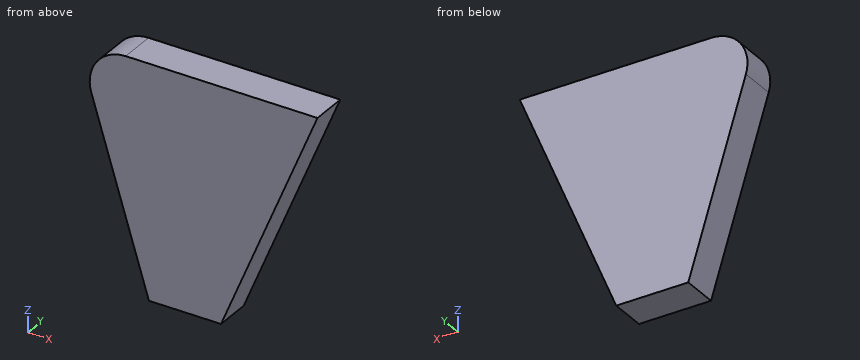
from build123d import *

# Parameters (mm, degrees)
F0_W     = 20
F0_H     = 32.335784
F1_DEPTH = 5
F3_DEPTH = 25
F4_R     = 5


with BuildPart() as f1:
    # F0 (on Front) → F1 (new body)
    with BuildSketch(Plane.XZ):
        with Locations((10, 16.167892)):
            Rectangle(F0_W, F0_H)
        Polygon((20, 32.335784), (20, 0), (33.39392, 32.335784), align=None)
    extrude(amount=F1_DEPTH)

    # F2 (on face) → F3 (cut)
    with BuildSketch(Plane.XZ.offset(5)):
        Polygon((10, 0), (0, 32.335784), (0, 0), align=None)
    extrude(amount=-F3_DEPTH, mode=Mode.SUBTRACT)

    # F4
    f4_edges = [f1.edges().sort_by_distance(p)[0] for p in [
        (0, -2.5, 32.335784),
    ]]
    fillet(f4_edges, radius=F4_R)


solid = f1.part
Can you work these out from the model? Positions are in its coordinate system, mm. Coordinates: 2 decimals unless noted, no trailing zeros. Write each loop counter-clockwise with the first axis right and the second up, starting at its lowest first coordinate (ties: lowest second). Pieces come first, ordered by that corner, then holes. Notation, with made-up numbers: (7, 88) - (32, 88) arc R16 ccw to (32, 118) - close; hole circle Ø5 at (-21, 61). An arc over 180 degrees is marked (long way). Return JSON: item names as keys, results as strings. Group by question number.
Item 1: If we section it at B-B (z = 12.5): Write out the boundary of the cut face in (x, y), then the cut area to 3 significant figures.
Item 2: If we section it at A-A (y = -1.5): Write out the boundary of the cut face in (x, z), then the cut area to 3 significant figures.
Item 3: If we section it at C-C (x = 4): Write out the boundary of the cut face in (y, z), then the cut area to 3 significant figures.
Item 4: Please list where these lines run through material, in increasing order: probe 1 along X at (y, z) = (-1.1, 12.5); probe 2 along X at (y, z) = (-3.95, 9); probe 3 along Z at (x, y) = (29.5, -0.85).
Return value:
{
 "1": {"outline": "(6.13, -5) - (25.18, -5) - (25.18, 0) - (6.13, 0) - close", "area": "95.2 mm^2"},
 "2": {"outline": "(2, 25.86) - (10, 0) - (20, 0) - (33.39, 32.34) - (6.78, 32.34) arc R5 ccw to start", "area": "691 mm^2"},
 "3": {"outline": "(-5, 19.4) - (0, 19.4) - (0, 31.49) - (-5, 31.49) - close", "area": "60.5 mm^2"},
 "4": {"probe 1": "x = 6.13 to 25.18", "probe 2": "x = 7.22 to 23.73", "probe 3": "z = 22.94 to 32.34"}
}
